Design review of the part built by this model. Coordinates are the model's own, in mm. Coordinates: 2 decimals unless noted, no trailing zeros. Order: outer loops, then holes, each group sorted by start corner. A loop starts at its lowest first (then second) coordinate and runs counter-clockwise, first axis right, second up. Notation, with made-up numbers: (-28, -35) -> (-19, -35) arc R7 ccw to (-19, -28) -> close; hole circle Ø6 at (23, 63.25). An arc over 180 degrees is marked (long way). Use a Markdown table: item, result. Add a question column.
Q1. Insertion check: pin 1 (17 mm diameter, centred on y = 177.8, z = 0, fed in from -X); pin 2 (22 mm diameter, centred on y = -177.8, z = 0, fed in from -X). Each pin has a flat end and moves straight along its axis. Give the tip position at first contact, or say it passes through.
Q2. Wall thickness on probe 1 along Y at (x, z) = (-2.5, 0) (3 decimals); probe 2 along Y at (x, z) = (5.5, 8.5); probe 3 along Z at (x, y) = (5.5, -175.5): over which ranges is each line inside the solid? List them lowest first.
Q3. Add section B-B (y = -177.8). State the section outline as (x, z) points (3 decimals).
Q4. Add section C-C (x = 1). State the section outline as (y, z) points (3 decimals), then the cut area to 3 significant figures.
Q5. Add section A-A (z = 0). State the section outline as (x, y) points (3 decimals).
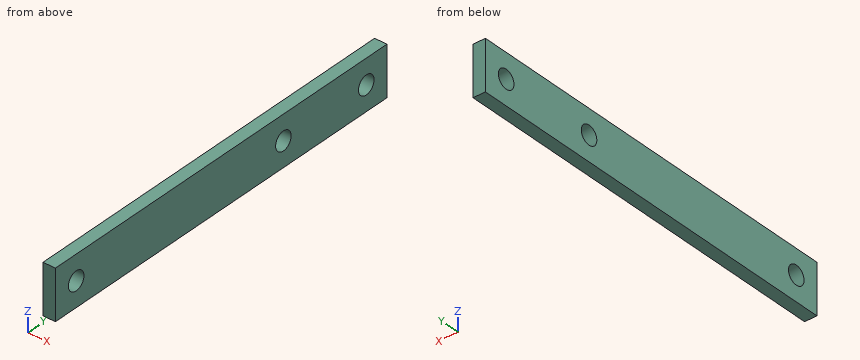
from build123d import *

# Parameters (mm, degrees)
SKETCH1_W           = 50.8
SKETCH1_H           = 406.4
BOSS_EXTRUDE1_DEPTH = 6.35
CUT_EXTRUDE1_REACH  = 14.7
SKETCH2_R           = 9.525


with BuildPart() as part:
    # Sketch1 → Boss-Extrude1 (new body, symmetric)
    with BuildSketch(Plane(origin=(0, 0, 0), x_dir=(0, 0, -1), z_dir=(1, 0, 0))):
        Rectangle(SKETCH1_W, SKETCH1_H)
    extrude(amount=BOSS_EXTRUDE1_DEPTH, both=True)

    # Sketch2 → Cut-Extrude1 (cut, up to next)
    with BuildSketch(Plane(origin=(6.35, 0, 0), x_dir=(0, 0, -1), z_dir=(1, 0, 0)), mode=Mode.PRIVATE) as cut_extrude1_sk1:
        with Locations((0, 177.8)):
            Circle(SKETCH2_R)
    cut_extrude1_tool1 = extrude(cut_extrude1_sk1.sketch, amount=-CUT_EXTRUDE1_REACH, mode=Mode.PRIVATE) & part.part
    add(cut_extrude1_tool1.solids().sort_by_distance((6.35, 177.8, 0))[0], mode=Mode.SUBTRACT)
    # Sketch2 → Cut-Extrude1 (cut, up to next)
    with BuildSketch(Plane(origin=(6.35, 0, 0), x_dir=(0, 0, -1), z_dir=(1, 0, 0)), mode=Mode.PRIVATE) as cut_extrude1_sk2:
        with Locations((0, -177.8)):
            Circle(SKETCH2_R)
    cut_extrude1_tool2 = extrude(cut_extrude1_sk2.sketch, amount=-CUT_EXTRUDE1_REACH, mode=Mode.PRIVATE) & part.part
    add(cut_extrude1_tool2.solids().sort_by_distance((6.35, -177.8, 0))[0], mode=Mode.SUBTRACT)
    # Sketch2 → Cut-Extrude1 (cut, up to next)
    with BuildSketch(Plane(origin=(6.35, 0, 0), x_dir=(0, 0, -1), z_dir=(1, 0, 0)), mode=Mode.PRIVATE) as cut_extrude1_sk3:
        with Locations((0, 76.2)):
            Circle(SKETCH2_R)
    cut_extrude1_tool3 = extrude(cut_extrude1_sk3.sketch, amount=-CUT_EXTRUDE1_REACH, mode=Mode.PRIVATE) & part.part
    add(cut_extrude1_tool3.solids().sort_by_distance((6.35, 76.2, 0))[0], mode=Mode.SUBTRACT)


solid = part.part
Established:
| question | item | result |
|---|---|---|
| 1 | pin 1 | through |
| 1 | pin 2 | x = -6.35 |
| 2 | probe 1 | -203.2 to -187.325, -168.275 to 66.675, 85.725 to 168.275, 187.325 to 203.2 |
| 2 | probe 2 | -203.2 to -182.1, -173.5 to 71.9, 80.5 to 173.5, 182.1 to 203.2 |
| 2 | probe 3 | -25.4 to -9.24, 9.24 to 25.4 |
| 3 | outline | (-6.35, -25.4) -> (6.35, -25.4) -> (6.35, -9.525) -> (-6.35, -9.525) -> close; (-6.35, 9.525) -> (6.35, 9.525) -> (6.35, 25.4) -> (-6.35, 25.4) -> close |
| 4 | outline | (-203.2, -25.4) -> (203.2, -25.4) -> (203.2, 25.4) -> (-203.2, 25.4) -> close; hole circle Ø19.05 at (-177.8, 0); hole circle Ø19.05 at (76.2, 0); hole circle Ø19.05 at (177.8, 0) |
| 4 | area | 19,800 mm^2 |
| 5 | outline | (-6.35, -203.2) -> (6.35, -203.2) -> (6.35, -187.325) -> (-6.35, -187.325) -> close; (-6.35, -168.275) -> (6.35, -168.275) -> (6.35, 66.675) -> (-6.35, 66.675) -> close; (-6.35, 85.725) -> (6.35, 85.725) -> (6.35, 168.275) -> (-6.35, 168.275) -> close; (-6.35, 187.325) -> (6.35, 187.325) -> (6.35, 203.2) -> (-6.35, 203.2) -> close |
